Geometry: final body of the model. Coordinates: model frame, mm. A direction names the side the tool comes from. Coordinates: 2 decimals unless noted, no trailing zeros. Write each loop counter-clockwise with the first axis right and the second up, starting at its lowest first coordinate (ties: lowest second). Pieces come first, ordered by that corner, then holes. Notation, with made-up numbers: (10.5, 85) - (57.5, 85) arc R23 ccw to (57.5, 120) - close; hole circle Ø6 at (48.5, 31.25). An arc over 180 degrees is marked (long way). Put each result on its own line as item: value.
```python
from build123d import *

# Parameters (mm, degrees)
F1_DEPTH      = 7.5
F1_DEPTH_BACK = 7.5
F2_R          = 2.5
F3_DEPTH      = 15.001
F4_R          = 1


with BuildPart() as f1:
    # F0 (on Front) → F1 (new body, two sides)
    with BuildSketch(Plane.XZ) as f1_sk:
        Polygon((36, 5), (-40, 5), (-40, -14), (-30, -14), (-30, 0), (0, 0), (0, -14), (36, -14), align=None)
    extrude(amount=F1_DEPTH)
    extrude(f1_sk.sketch, amount=-F1_DEPTH_BACK)

    # F2 (on face) → F3 (cut, through all)
    with BuildSketch(Plane.XZ.offset(7.5)):
        with Locations((36, 1.5)):
            Circle(F2_R)
        with Locations((36, -4.5)):
            Circle(F2_R)
        with Locations((36, -10.5)):
            Circle(F2_R)
    extrude(amount=-F3_DEPTH, mode=Mode.SUBTRACT)

    # F4
    f4_edges = [f1.edges().sort_by_distance(p)[0] for p in [
        (-30, 0, -14),
        (0, 0, -14),
    ]]
    fillet(f4_edges, radius=F4_R)


solid = f1.part
```
1. Section query C-C (x = -26). Return loops of the section in (y, z).
Answer below:
outline: (-7.5, 0) - (7.5, 0) - (7.5, 5) - (-7.5, 5) - close
2. Section query A-A (z = -10.5). Return loops of the section in (x, y), then the cut area to 4 significant figures.
Answer below:
outline: (-40, -7.5) - (-30, -7.5) - (-30, 7.5) - (-40, 7.5) - close; (0, -7.5) - (33.5, -7.5) - (33.5, 7.5) - (0, 7.5) - close
area: 652.5 mm²
3. Section query B-B (y = -4.5). Return loops of the section in (x, z), then the cut area to 3 significant figures.
Answer below:
outline: (-40, -14) - (-31, -14) arc R1 ccw to (-30, -13) - (-30, 0) - (0, 0) - (0, -13) arc R1 ccw to (1, -14) - (36, -14) - (36, -13) arc R2.5 cw to (36, -8) - (36, -7) arc R2.5 cw to (36, -2) - (36, -1) arc R2.5 cw to (36, 4) - (36, 5) - (-40, 5) - close
area: 994 mm²
4. Mould query, pull axis X, two halves, no side actions, for faces 1 (the flat face through (-15, 0, 0)), 2 (the flat face through (-1, 0, 5)), 3 (the cylindrical face through (33.5, -0.1, -4.4)), 4 (the flat face through (-30, 0, -7)). Classes: +X half, -X half, draft (parallel to the pull), parting line (faces both ways), or undercut.
Answer below:
face 1: undercut
face 2: draft
face 3: +X half
face 4: undercut
5. Section query D-D (z = 1.5). Return loops of the section in (x, y), then the cut area to 3 significant figures.
Answer below:
outline: (-40, -7.5) - (33.5, -7.5) - (33.5, 7.5) - (-40, 7.5) - close
area: 1,100 mm²
6. Ray query, probe 1 along X at (y, z) = (2.75, -7.75); probe 2 along Z at (x, y) = (-5.5, 0); probe 3 along X at (y, z) = (-2.75, -9.75). Return the intervals inside material, ascending. Write a range as from..to.
Answer below:
probe 1: x = -40..-30, 0..36
probe 2: z = 0..5
probe 3: x = -40..-30, 0..33.62
7. Set-up query: faces 5 (the flat face through (-36, 0, -14)), 6 (the flat face through (0, 0, -6)). Return all of +Z, -Z, +X, -X, +Y, -Y with unobstructed straight access to the full face (end or side cutting, diameter ignored); none if empty.
Answer below:
face 5: -Z, +X, -X, +Y, -Y
face 6: -Z, +Y, -Y
